Read the model definition and answer for the solid it produces. Units are mm, in the model's axes. Face numbers are marked on the shaded views. A direction names the side the tool comes from. Round coordinates to 2 decimals unless told otherwise and drop trailing zeros. Loops run counter-clockwise (first coordinate to the right, second up) from the corner with the lowest first, then second, coordinate; pieces in that order, holes last. Notation, with made-up numbers: (0.25, -37) - (9.25, -37) arc R13 ccw to (9.25, -30) - close; hole circle Ø8 at (70.5, 50). An arc over 180 degrees is marked (long way). Use CSV: the item, a comma, the result in double quotes. Start each with the question number.
1. Find section B-B (y = -9). Give the vertices of the cut face in (x, z).
2. A tool of negligible diameter and unlimited length cuts with its end or side. For the marked faces 4, 5 and 6, from which of +Z, -Z, +X, -X, +Y, -Y can it reach the whole face along a straight path? Write none if from no direction.
3. Find section D-D (x = 8). Give the vertices of the cut face in (y, z).
4. Find section A-A (z = 9). Give the vertices of the cut face in (x, y), and give its area (3 significant figures).
5. Find section C-C (x = -17). Give the vertices of the cut face in (y, z), and give its area (3 significant figures).
6. Given pin 1 Ø14.5 at (x, y) = (19, 12.5) entering from +Z; pin 2 Ø3 at (x, y) = (-7.5, 21.5) entering from -Z; pin 3 Ø1.5 at (x, y) = (2, 21.5) entering from +Z, each flat-ended and moving along its own axis, determine where each tip first touches the part or whether it passes through.
7. Consider line 1 along X through (y, z) = (-21, 33); line 2 along Y through (x, z) = (-4, 121). Determine where each line is inside the solid, lowest interval first.
8. Determine the mould class of the marked faces 1, 2 and 3 for opening direction X: +X half, -X half, draft (parallel to the pull), parting line (faces both ways), or undercut.
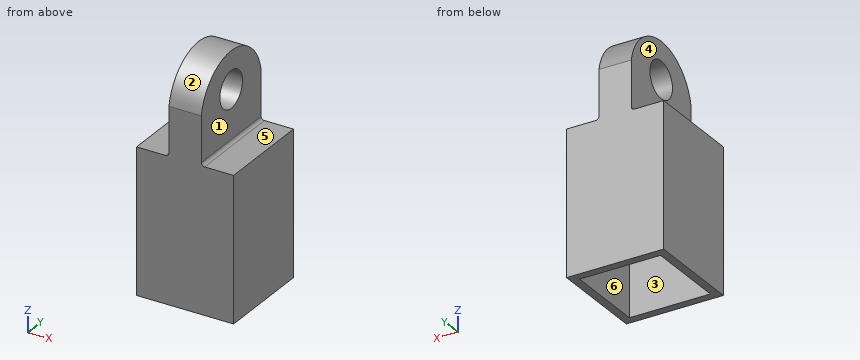
from build123d import *

# Parameters (mm, degrees)
SKETCH2_W           = 60
SKETCH2_H           = 60
BOSS_EXTRUDE1_DEPTH = 89
SKETCH3_W           = 20
SKETCH3_H           = 60
BOSS_EXTRUDE2_DEPTH = 30
BOSS_EXTRUDE3_DEPTH = 20
FILLET1_R           = 2
SKETCH7_W           = 50
SKETCH7_H           = 50
CUT_EXTRUDE1_DEPTH  = 81
SKETCH8_R           = 11.35
CUT_EXTRUDE2_DEPTH  = 153.570263572


with BuildPart() as part:
    # Sketch2 → Boss-Extrude1 (new body)
    with BuildSketch(Plane.XY):
        Rectangle(SKETCH2_W, SKETCH2_H)
    extrude(amount=BOSS_EXTRUDE1_DEPTH)

    # Sketch3 → Boss-Extrude2 (add)
    with BuildSketch(Plane.XY.offset(89)):
        Rectangle(SKETCH3_W, SKETCH3_H)
    extrude(amount=BOSS_EXTRUDE2_DEPTH)

    # Sketch4 → Boss-Extrude3 (add)
    with BuildSketch(Plane(origin=(10, 0, 0), x_dir=(0, 0, -1), z_dir=(1, 0, 0))):
        with BuildLine():
            Line((-119, -30), (-119, 30))
            ThreePointArc((-119, 30), (-144.144668047, 0), (-119, -30))
        make_face()
    extrude(amount=-BOSS_EXTRUDE3_DEPTH)

    # Fillet1
    fillet1_edges = [part.edges().sort_by_distance(p)[0] for p in [
        (-10, 0, 89),
        (10, 0, 89),
    ]]
    fillet(fillet1_edges, radius=FILLET1_R)

    # Sketch7 → Cut-Extrude1 (cut)
    with BuildSketch(Plane(origin=(0, 0, 0), x_dir=(-1, 0, 0), z_dir=(0, 0, -1))):
        Rectangle(SKETCH7_W, SKETCH7_H)
    extrude(amount=-CUT_EXTRUDE1_DEPTH, mode=Mode.SUBTRACT)

    # Sketch8 → Cut-Extrude2 (cut, through all)
    with BuildSketch(Plane.ZY.offset(10)):
        with Locations((121, 0)):
            Circle(SKETCH8_R)
    extrude(amount=-CUT_EXTRUDE2_DEPTH, mode=Mode.SUBTRACT)


solid = part.part
Filled sheet:
1,outline,"(-30, 0) - (-25, 0) - (-25, 81) - (25, 81) - (25, 0) - (30, 0) - (30, 89) - (12, 89) arc R2 cw to (10, 91) - (10, 114.08) - (-10, 114.08) - (-10, 91) arc R2 cw to (-12, 89) - (-30, 89) - close; (-10, 127.92) - (10, 127.92) - (10, 142.79) - (-10, 142.79) - close"
2,face 4,"+Z, -X, +Y, -Y"
2,face 5,"+Z, +X, +Y, -Y"
2,face 6,"-Z"
3,outline,"(-30, 0) - (-25, 0) - (-25, 81) - (25, 81) - (25, 0) - (30, 0) - (30, 119) arc R30.47 ccw to (-30, 119) - close; hole circle Ø22.7 at (0, 121)"
4,outline,"(-30, -30) - (30, -30) - (30, 30) - (-30, 30) - close; hole (-25, -25) - (25, -25) - (25, 25) - (-25, 25) - close"
4,area,"1,100 mm²"
5,outline,"(-30, 0) - (-25, 0) - (-25, 81) - (25, 81) - (25, 0) - (30, 0) - (30, 89) - (-30, 89) - close"
5,area,"1,290 mm²"
6,pin 1,"stops at z = 89.02"
6,pin 2,"stops at z = 81"
6,pin 3,"stops at z = 135.99"
7,line 1,"x = -30 to -25, 25 to 30"
7,line 2,"y = -29.58 to -11.35, 11.35 to 29.58"
8,face 1,"+X half"
8,face 2,"draft"
8,face 3,"undercut"
